from build123d import *

# Parameters (mm, degrees)
BOSS_EXTRUDE2_DEPTH = 12.7
FILLET2_R           = 2.5


with BuildPart() as part:
    # Sketch1 → Boss-Extrude2 (new body)
    with BuildSketch(Plane.XY):
        Polygon((0, 0), (-611.632, 0), (-611.632, 607.568), (0, 607.568), (0, 587.480907233), (-209.519092864, 587.480907233), (-209.519092864, 384.280907233), (0, 384.280907233), align=None)
        with BuildLine():
            Line((-5, 10.5), (-5, 9.5))
            ThreePointArc((-5, 9.5), (-5.732233047, 7.732233047), (-7.5, 7))
            Line((-7.5, 7), (-12.5, 7))
            ThreePointArc((-12.5, 7), (-14.267766953, 7.732233047), (-15, 9.5))
            Line((-15, 9.5), (-15, 10.5))
            ThreePointArc((-15, 10.5), (-14.267766953, 12.267766953), (-12.5, 13))
            Line((-12.5, 13), (-7.5, 13))
            ThreePointArc((-7.5, 13), (-5.732233047, 12.267766953), (-5, 10.5))
        make_face(mode=Mode.SUBTRACT)
        with BuildLine():
            Line((-596.63, 10.5), (-596.63, 9.5))
            ThreePointArc((-596.63, 9.5), (-597.362233047, 7.732233047), (-599.13, 7))
            Line((-599.13, 7), (-604.13, 7))
            ThreePointArc((-604.13, 7), (-605.897766953, 7.732233047), (-606.63, 9.5))
            Line((-606.63, 9.5), (-606.63, 10.5))
            ThreePointArc((-606.63, 10.5), (-605.897766953, 12.267766953), (-604.13, 13))
            Line((-604.13, 13), (-599.13, 13))
            ThreePointArc((-599.13, 13), (-597.362233047, 12.267766953), (-596.63, 10.5))
        make_face(mode=Mode.SUBTRACT)
        with BuildLine():
            Line((-596.63, 598.07), (-596.63, 597.07))
            ThreePointArc((-596.63, 597.07), (-597.362233047, 595.302233047), (-599.13, 594.57))
            Line((-599.13, 594.57), (-604.13, 594.57))
            ThreePointArc((-604.13, 594.57), (-605.897766953, 595.302233047), (-606.63, 597.07))
            Line((-606.63, 597.07), (-606.63, 598.07))
            ThreePointArc((-606.63, 598.07), (-605.897766953, 599.837766953), (-604.13, 600.57))
            Line((-604.13, 600.57), (-599.13, 600.57))
            ThreePointArc((-599.13, 600.57), (-597.362233047, 599.837766953), (-596.63, 598.07))
        make_face(mode=Mode.SUBTRACT)
        with BuildLine():
            Line((-5, 598.07), (-5, 597.07))
            ThreePointArc((-5, 597.07), (-5.732233047, 595.302233047), (-7.5, 594.57))
            Line((-7.5, 594.57), (-12.5, 594.57))
            ThreePointArc((-12.5, 594.57), (-14.267766953, 595.302233047), (-15, 597.07))
            Line((-15, 597.07), (-15, 598.07))
            ThreePointArc((-15, 598.07), (-14.267766953, 599.837766953), (-12.5, 600.57))
            Line((-12.5, 600.57), (-7.5, 600.57))
            ThreePointArc((-7.5, 600.57), (-5.732233047, 599.837766953), (-5, 598.07))
        make_face(mode=Mode.SUBTRACT)
    extrude(amount=BOSS_EXTRUDE2_DEPTH)

    # Fillet2
    fillet2_edges = [part.edges().sort_by_distance(p)[0] for p in [
        (0, 0, 6.35),
        (-611.632, 0, 6.35),
        (-611.632, 607.568, 6.35),
        (0, 607.568, 6.35),
    ]]
    fillet(fillet2_edges, radius=FILLET2_R)


solid = part.part
For this review, take the finished solid that the model builds, in its own axes (mm). Give positions to 0.01 mm unless a question says otherwise; leave off trailing zeros. Loops run counter-clockwise (first coordinate to the right, second up) from the corner with the lowest first, then second, coordinate; pieces in that order, holes last.
Item 1: For line 1 along Y through (x, z) = (-170, 9.5); line 2 along X through (y, z) = (538.5, 10), list the stretches that pass through material, from the lowest coordinate up.
Item 2: Take a section at B-B, the plane z = 5.5. Give the number of separate pieces and of enclosed holes in the cut face, and give its area (3 significant figures).
Item 3: Insertion check: pin 1 (4 mm diameter, centred on y = 526, z = 6.5, fed in from +X). The pin has a flat end and moves straight along its axis. Give the tip position at first contact, or say it passes through.
Item 4: Take a section at A-A, the plane x = -98.5. State the section outline as (y, z) points, and give its area (3 significant figures).
Item 5: Take a section at C-C, the plane y = 428.5. State the section outline as (x, z) points.
Calculated:
1. line 1: y = 0 to 384.28, 587.48 to 607.57
1. line 2: x = -611.63 to -209.52
2. separate pieces: 1
2. enclosed holes: 4
2. area: 329,000 mm2
3. pin 1: stops at x = -209.52
4. outline: (0, 0) - (384.28, 0) - (384.28, 12.7) - (0, 12.7) - close; (587.48, 0) - (607.57, 0) - (607.57, 12.7) - (587.48, 12.7) - close
4. area: 5,140 mm2
5. outline: (-611.63, 0) - (-209.52, 0) - (-209.52, 12.7) - (-611.63, 12.7) - close
